```python
from build123d import *

# Parameters (mm, degrees)
SKETCH1_W           = 20
SKETCH1_H           = 20
SKETCH1_R           = 3
BOSS_EXTRUDE1_DEPTH = 19.63
CUT_EXTRUDE1_DEPTH  = 26
CUT_EXTRUDE2_DEPTH  = 26
CHAMFER1_SIZE       = 0.25
CHAMFER2_SIZE       = 0.25


with BuildPart() as part:
    # Sketch1 → Boss-Extrude1 (new body)
    with BuildSketch(Plane.XY):
        Rectangle(SKETCH1_W, SKETCH1_H)
        Circle(SKETCH1_R, mode=Mode.SUBTRACT)
    extrude(amount=BOSS_EXTRUDE1_DEPTH)

    # Sketch2 → Cut-Extrude1 (cut)
    with BuildSketch(Plane(origin=(0, 0, 0), x_dir=(-1, 0, 0), z_dir=(0, 0, -1))):
        Polygon((-6, 8.5), (-4.5, 10), (-7.5, 10), align=None)
        Polygon((-1.5, 10), (0, 8.5), (1.5, 10), align=None)
        Polygon((7.5, 10), (4.5, 10), (6, 8.5), align=None)
    extrude(amount=-CUT_EXTRUDE1_DEPTH, mode=Mode.SUBTRACT)

    # Sketch3 → Cut-Extrude2 (cut)
    with BuildSketch(Plane(origin=(-10, 0, 10), x_dir=(0, 0, -1), z_dir=(1, 0, 0))):
        Polygon((7.5, 10), (4.5, 10), (6, 8.5), align=None)
        Polygon((-1.5, 10), (0, 8.5), (1.5, 10), align=None)
        Polygon((-6, 8.5), (-4.5, 10), (-7.5, 10), align=None)
    extrude(amount=CUT_EXTRUDE2_DEPTH, mode=Mode.SUBTRACT)

    # Chamfer1
    chamfer1_edges = [part.edges().sort_by_distance(p)[0] for p in [
        (-3, 0, 0),
    ]]
    chamfer(chamfer1_edges, length=CHAMFER1_SIZE)

    # Chamfer2
    chamfer2_edges = [part.edges().sort_by_distance(p)[0] for p in [
        (-3, 0, 19.63),
    ]]
    chamfer(chamfer2_edges, length=CHAMFER2_SIZE)


solid = part.part
```
CAD build for the part. Positions are in the model's coordinates, mm. A direction names the side the tool comes from. Give positions to 0.01 mm unless a question says otherwise; leave off trailing zeros. Order: outer loops, then holes, each group sorted by start corner. A loop starts at its lowest first (then second) coordinate and runs counter-clockwise, first axis right, second up.
(1) Drill centre lines: L1, parallel to X at y = 1.5, z = 18.25; L2, parallel to Y at x = 2.75, z = 4.5; L3, parallel to Y at x = 2.25, z = 7.75. Where is each one in solid material? Low to high.
(2) Saw through at B-B, the plane y = 0. Give the cut face in (x, z), then the cut area to 3 significant figures.
(3) Saw through at A-A, the plane z = 17. Give the cut face in (x, y).
(4) Saw through at D-D, the plane z = 12.25. Give the cut face in (x, y).
(5) Flat gauge pins, fed straight in: pin 1 (1 mm diameter, centred on x = -6.5, z = 17, fed in from +Y); pin 2 (1 mm diameter, centred on x = 6, z = 15.5, fed in from +Y). Where does each tip first touch, or does it go through?
(6) Tool access for faces 4 (the flat face through (0.8, 9.3, 1.5)), 5 (the flat face through (8.4, 9.3, 16.8)), 6 (the flat face through (3, 10, 7)): list every direction of +Z, -Z, +X, -X, +Y, -Y with a clear straight run to the whole face (end or side of a thin tool).
(7) Saw through at C-C, the plane x = -8.25. Give the cut face in (y, z), then the cut area to 3 significant figures.
(8) Mould opens along Z. For faces 1 (the flat face through (-3, 9.1, 16.6)), 2 (the flat face through (0, -4, 0)), 3 (the flat face through (-3, 10, 7)) say: released by +Z, released by -Z, zero draft, split by the parting line, or undercut.
Results found:
1. L1: x = -10 to -2.6, 2.6 to 10
1. L2: y = -10 to -1.2, 1.2 to 9
1. L3: y = -10 to -1.98, 1.98 to 10
2. outline: (-10, 0) - (-3.25, 0) - (-3, 0.25) - (-3, 19.38) - (-3.25, 19.63) - (-10, 19.63) - close; (3, 0.25) - (3.25, 0) - (10, 0) - (10, 19.63) - (3.25, 19.63) - (3, 19.38) - close
2. area: 275 mm2
3. outline: (-10, -10) - (10, -10) - (10, 9.5) - (7, 9.5) - (6, 8.5) - (5, 9.5) - (1, 9.5) - (0, 8.5) - (-1, 9.5) - (-5, 9.5) - (-6, 8.5) - (-7, 9.5) - (-10, 9.5) - close; hole circle Ø6 at (0, 0)
4. outline: (-10, -10) - (10, -10) - (10, 10) - (7.5, 10) - (6, 8.5) - (4.5, 10) - (1.5, 10) - (0, 8.5) - (-1.5, 10) - (-4.5, 10) - (-6, 8.5) - (-7.5, 10) - (-10, 10) - close; hole circle Ø6 at (0, 0)
5. pin 1: stops at y = 9.5
5. pin 2: stops at y = 9
6. face 4: +Z, -Z, +Y
6. face 5: +X, -X, +Y
6. face 6: +Z, -Z, +X, -X, +Y
7. outline: (-10, 0) - (10, 0) - (10, 2.5) - (8.5, 4) - (10, 5.5) - (10, 8.5) - (8.5, 10) - (10, 11.5) - (10, 14.5) - (8.5, 16) - (10, 17.5) - (10, 19.63) - (-10, 19.63) - close
7. area: 386 mm2
8. face 1: undercut
8. face 2: released by -Z
8. face 3: zero draft
